from build123d import *

# Parameters (mm, degrees)
SKETCH1_R           = 1.778
SKETCH1_R_2         = 9.525
BOSS_EXTRUDE1_DEPTH = 6.35
FILLET1_R           = 3.81
FILLET2_R           = 2.54


with BuildPart() as part:
    # Sketch1 → Boss-Extrude1 (new body)
    with BuildSketch(Plane(origin=(0, 0, 0), x_dir=(1, 0, 0), z_dir=(0, 1, 0))):
        Polygon((-25.4, 38.1), (-25.4, 44.45), (-50.8, 44.45), (-50.8, -44.45), (-25.4, -44.45), (-25.4, -38.1), (0, -38.1), (25.4, -38.1), (25.4, -44.45), (50.8, -44.45), (50.8, 0), (50.8, 44.45), (25.4, 44.45), (25.4, 38.1), align=None)
        Polygon((31.75, -34.29), (0, -34.29), (-31.75, -34.29), (-14.867118492, -17.407118492), (14.867118492, -17.407118492), align=None, mode=Mode.SUBTRACT)
        with Locations(Location((-15.24, -15.24, 0), (0, 0, 270))):
            Circle(SKETCH1_R, mode=Mode.SUBTRACT)
        with Locations(Location((15.24, -15.24, 0), (0, 0, 270))):
            Circle(SKETCH1_R, mode=Mode.SUBTRACT)
        with Locations(Location((-15.24, 15.24, 0), (0, 0, 270))):
            Circle(SKETCH1_R, mode=Mode.SUBTRACT)
        with Locations(Location((15.24, 15.24, 0), (0, 0, 270))):
            Circle(SKETCH1_R, mode=Mode.SUBTRACT)
        Polygon((40.64, 31.75), (40.64, 0), (40.64, -31.75), (23.757118492, -14.867118492), (23.757118492, 0), (23.757118492, 14.867118492), align=None, mode=Mode.SUBTRACT)
        Polygon((-40.64, -25.4), (-40.64, 38.1), (-23.757118492, 21.217118492), (-23.757118492, -8.517118492), align=None, mode=Mode.SUBTRACT)
        Polygon((-31.75, 34.29), (31.75, 34.29), (14.867118492, 17.407118492), (-14.867118492, 17.407118492), align=None, mode=Mode.SUBTRACT)
        with Locations(Location((0, 0, 0), (0, 0, 270))):
            Circle(SKETCH1_R_2, mode=Mode.SUBTRACT)
    extrude(amount=BOSS_EXTRUDE1_DEPTH)

    # Fillet1
    fillet1_edges = [part.edges().sort_by_distance(p)[0] for p in [
        (14.867118492, 3.175, -17.407118492),
        (-14.867118492, 3.175, -17.407118492),
        (14.867118492, 3.175, 17.407118492),
        (-14.867118492, 3.175, 17.407118492),
        (23.757118492, 3.175, -14.867118492),
        (23.757118492, 3.175, 14.867118492),
        (-23.757118492, 3.175, 8.517118492),
        (-23.757118492, 3.175, -21.217118492),
    ]]
    fillet(fillet1_edges, radius=FILLET1_R)

    # Fillet2
    fillet2_edges = [part.edges().sort_by_distance(p)[0] for p in [
        (31.75, 3.175, -34.29),
        (-31.75, 3.175, -34.29),
        (-31.75, 3.175, 34.29),
        (31.75, 3.175, 34.29),
        (40.64, 3.175, -31.75),
        (40.64, 3.175, 31.75),
        (-40.64, 3.175, 25.4),
        (-40.64, 3.175, -38.1),
    ]]
    fillet(fillet2_edges, radius=FILLET2_R)


solid = part.part
Verification items for the finished model (mm, model axes). A direction names the side the tool comes from. Round coordinates to 2 decimals unless told otherwise and drop trailing zeros. Loops run counter-clockwise (first coordinate to the right, second up) from the corner with the lowest first, then second, coordinate; pieces in that order, holes last. Notation, with made-up numbers: (33.5, -21) - (48.5, -21) arc R21 ccw to (48.5, -1) - close; hole circle Ø1 at (-3.5, -36.5). An arc over 180 degrees is marked (long way). Use a Markdown table: item, result. Add a question column.
1. Gauge pin test, flat ends, axial feed: pin 1 (3 mm diameter, centred on x = -12, y = 4.5, fed in from +Z); pin 2 (2 mm diameter, centred on x = -15.24, z = -15.24, fed in from -Y); pin 3 (3 mm diameter, centred on x = 1, y = 3.5, fed in from -Z). Record the tip position at first contact, or that the pin passes through.
2. Section check D-D, the plane y = 4. Give the number of separate pieces and of enclosed holes in the cut face, plus the area to 3 significant figures.
3. Thickness scan on probe 1 along X at (y, z) = (3.75, 0) (3 decimals); probe 2 along X at (y, z) = (1, 31.5); probe 3 along Z at (x, y) = (6, 1.5). Record the ranges inside material, lowest first. Write a range as [from, to].
4. Section check A-A, the plane z = 0. Record the boundary of the cut face in (x, y) (3 decimals).
5. Section check B-B, the plane x = 31.5. Record the boundary of the cut face in (y, z).
6. Access from +Z, -Z, +X, -X, +Y, -Y to the whole of each face (thin tool, end or side, straight path). Record for faces 1 (the face through (25.4, 3, 41)), 2 (the face through (-25.4, 3, -41)), 3 (the face through (0, 3, 17.407)).
7. Section check C-C, the plane x = -4.5. Record the boundary of the cut face in (y, z), plus the area to 3 significant figures.
Checks:
| question | item | result |
|---|---|---|
| 1 | pin 1 | stops at z = 38.1 |
| 1 | pin 2 | passes through |
| 1 | pin 3 | stops at z = -38.1 |
| 2 | separate pieces | 1 |
| 2 | enclosed holes | 9 |
| 2 | area | 4,980 mm^2 |
| 3 | probe 1 | x = [-50.8, -40.64], [-23.757, -9.525], [9.525, 23.757], [40.64, 50.8] |
| 3 | probe 2 | x = [-50.8, -28.15], [28.15, 50.8] |
| 3 | probe 3 | z = [-38.1, -34.29], [-17.41, -7.4], [7.4, 17.41], [34.29, 38.1] |
| 4 | outline | (-50.8, 0) - (-40.64, 0) - (-40.64, 6.35) - (-50.8, 6.35) - close; (-23.757, 0) - (-9.525, 0) - (-9.525, 6.35) - (-23.757, 6.35) - close; (9.525, 0) - (23.757, 0) - (23.757, 6.35) - (9.525, 6.35) - close; (40.64, 0) - (50.8, 0) - (50.8, 6.35) - (40.64, 6.35) - close |
| 5 | outline | (0, -44.45) - (6.35, -44.45) - (6.35, -22.61) - (0, -22.61) - close; (0, 22.61) - (6.35, 22.61) - (6.35, 44.45) - (0, 44.45) - close |
| 6 | face 1 | +Z, +Y, -Y |
| 6 | face 2 | -Z, +Y, -Y |
| 6 | face 3 | +Y, -Y |
| 7 | outline | (0, -38.1) - (6.35, -38.1) - (6.35, -34.29) - (0, -34.29) - close; (0, -17.41) - (6.35, -17.41) - (6.35, -8.39) - (0, -8.39) - close; (0, 8.39) - (6.35, 8.39) - (6.35, 17.41) - (0, 17.41) - close; (0, 34.29) - (6.35, 34.29) - (6.35, 38.1) - (0, 38.1) - close |
| 7 | area | 163 mm^2 |
